CAD build for the part. Positions are in the model's coordinates, mm. Coordinates: 2 decimals unless noted, no trailing zeros. Loops run counter-clockwise (first coordinate to the right, second up) from the corner with the lowest first, then second, coordinate; pieces in that order, holes last. Notation, with made-up numbers: (43.5, -28.5) -> (81.5, -28.5) arc R27 ccw to (81.5, 8.5) -> close; hole circle Ø1 at (28, -35.5). An arc over 180 degrees is marked (long way). Return JSON: item names as keys, results as strings. Group by question number.
(1) Saw through at B-B on y = -20. Write the cut outline in (x, z), then the cut area to 3 significant figures.
(2) Saw through at A-A on y = 70. Write the cut outline in (x, z).
(3) Saw through at C-C on x = 52.5. Write the cut outline in (y, z), then the cut area to 3 significant figures.
(4) Probe L1, parallel to Y at x = 97.5, z = 1.6; L2, parallel to Y at x = 0, z = 1.8; L3, parallel to X at y = 67, z = 4.45. List the from-to ranges inside material, lowest first.
(5) Flat gauge pin, fed straight in: pin 1 Ø13.5 at (x, y) = (102.5, 70) entering from -Z. Where does the tip first touch, or does it go through?
```python
from build123d import *

# Parameters (mm, degrees)
SKETCH1_W            = 235
SKETCH1_H            = 160
BOSS_EXTRUDE1_DEPTH  = 5
M8_CLEARANCE_HOLE1_D = 8.4


with BuildPart() as part:
    # Sketch1 → Boss-Extrude1 (new body)
    with BuildSketch(Plane.XY):
        Rectangle(SKETCH1_W, SKETCH1_H)
    extrude(amount=BOSS_EXTRUDE1_DEPTH)

    # M8 Clearance Hole1 (through all)
    with Locations(Plane.XY.offset(5)):
        with Locations((-102.5, 70), (-97.5, -20), (-97.5, -60), (-52.5, 70), (0, 70), (52.5, 70), (102.5, 70), (97.5, -20), (97.5, -60)):
            Hole(M8_CLEARANCE_HOLE1_D / 2)


solid = part.part
```
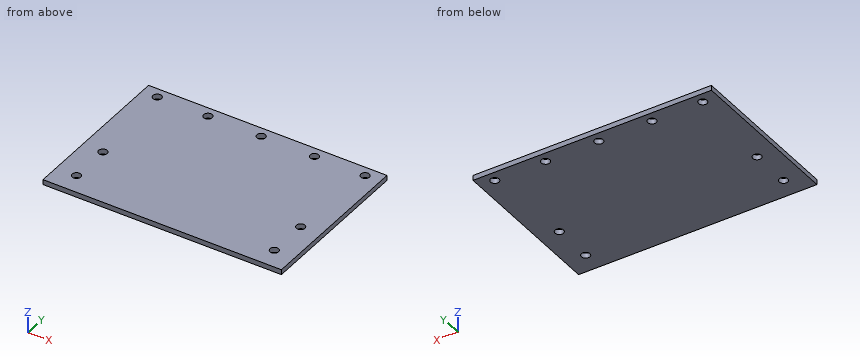
Geometry results:
{
 "1": {"outline": "(-117.5, 0) -> (-101.7, 0) -> (-101.7, 5) -> (-117.5, 5) -> close; (-93.3, 0) -> (93.3, 0) -> (93.3, 5) -> (-93.3, 5) -> close; (101.7, 0) -> (117.5, 0) -> (117.5, 5) -> (101.7, 5) -> close", "area": "1,090 mm²"},
 "2": {"outline": "(-117.5, 0) -> (-106.7, 0) -> (-106.7, 5) -> (-117.5, 5) -> close; (-98.3, 0) -> (-56.7, 0) -> (-56.7, 5) -> (-98.3, 5) -> close; (-48.3, 0) -> (-4.2, 0) -> (-4.2, 5) -> (-48.3, 5) -> close; (4.2, 0) -> (48.3, 0) -> (48.3, 5) -> (4.2, 5) -> close; (56.7, 0) -> (98.3, 0) -> (98.3, 5) -> (56.7, 5) -> close; (106.7, 0) -> (117.5, 0) -> (117.5, 5) -> (106.7, 5) -> close"},
 "3": {"outline": "(-80, 0) -> (65.8, 0) -> (65.8, 5) -> (-80, 5) -> close; (74.2, 0) -> (80, 0) -> (80, 5) -> (74.2, 5) -> close", "area": "758 mm²"},
 "4": {"L1": "-80 to -64.2, -55.8 to -24.2, -15.8 to 80", "L2": "-80 to 65.8, 74.2 to 80", "L3": "-117.5 to -105.44, -99.56 to -55.44, -49.56 to -2.94, 2.94 to 49.56, 55.44 to 99.56, 105.44 to 117.5"},
 "5": {"pin 1": "z = 0"}
}
